Geometry check sheet. Reference: the model listing, model coordinates, mm. A direction names the side the tool comes from. Give positions to 0.01 mm unless a question says otherwise; leave off trailing zeros. Write each loop counter-clockwise with the first axis right and the second up, starting at its lowest first coordinate (ties: lowest second). Pieces come first, ordered by that corner, then holes. Notation, with made-up numbers: M 64.25,30.5 L 110.25,30.5 A33 ccw 110.25,58.5 Z; hole C -25.5,82.5 d2. An arc over 180 degrees is marked long. Write each question's results on one line, items separated by ' | '.
Autodesk Inventor part; units mm, degrees
ref_plane "YZ Plane" through (0, 0, 0) normal (1, 0, 0) x (0, 1, 0)
ref_plane "XZ Plane" through (0, 0, 0) normal (0, 1, 0) x (-1, 0, 0)
ref_plane "XY Plane" through (0, 0, 0) normal (0, 0, 1) x (1, 0, 0)
ref_plane "Work Plane1" through (0, 46.8, 0) normal (0, 0, 1) x (-1, 0, 0)
sketch "Sketch2" plane through (0, 46.8, 0) normal (0, 0, 1) x (-1, 0, 0)
  spline S0 degree 3 number of poles 148
  spline S1 degree 3 number of poles 148
  line L0 (31.3425, -5.6798) -> (32.5946, -4.8031)
  line L1 (32.5946, -4.1553) -> (31.3425, -3.2786)
  line L2 (31.3425, -3.2786) -> (31.3425, -5.6037)
  line L3 (32.5946, -4.8031) -> (32.5946, -4.1553)
  line L4 (31.3425, 13.5614) -> (31.3425, -5.6037)
  line L5 (32.8425, -4.1071) -> (31.4425, -3.1268)
  line L6 (31.4425, -3.1268) -> (31.4425, -2.831)
  line L7 (31.4425, -2.831) -> (32.8425, -1.8994)
  line L8 (32.8425, -1.8994) -> (32.8425, -4.1071)
  point P0 (0, 46.8)
  point P1 (31.9686, -3.7169)
  point P2 (32.1425, -3.6169)
  point P3 (31.4425, -2.9789)
  dimension "d4" = 0
  dimension "d5" = 0.1
  dimension "d6" = 0.1
  dimension "d7" = 1.4
coil "Coil1" sketch "Sketch2" operation add axis through (-23.4, 35.1998, 0) along (0, -1, 0) pitch 3 turns 2.5 hand right contours L5 L6 L7 L8
sketch "Sketch3" plane through (0, 46.8, 0) normal (0, 0, 1) x (-1, 0, 0)
  line L0 (13.9575, 5.6006) -> (13.9575, 3.3929)
  line L1 (32.8425, -1.8994) -> (32.8425, -4.1071)
  line L2 (15.3575, 4.669) -> (13.9575, 5.6006)
  line L3 (13.9575, 5.6006) -> (11.9575, 5.6006)
  line L4 (11.9575, 5.6006) -> (11.9575, -1.1071)
  line L5 (11.9575, -1.1071) -> (13.9575, -1.1071)
  line L6 (13.9575, -1.1071) -> (13.9575, 5.6006)
  line L7 (11.9575, -1.1071) -> (16.9575, -1.1071)
  line L8 (16.9575, -1.1071) -> (16.9575, -3.1071)
  line L9 (16.9575, -3.1071) -> (11.9575, -3.1071)
  line L10 (11.9575, -3.1071) -> (11.9575, -1.1071)
  line L11 (23.4, 56.7814) -> (23.4, -13.0885)
  point P0 (0, 46.8)
  dimension "d16" = 2
  dimension "d17" = 5
  dimension "d18" = 2
revolve "Revolution2" add sketch "Sketch3" angle 360 about axis through (-23.4, 35.1998, 0) along (0, 1, 0)
fillet "Fillet1" radius 1 4 edges at (-34.8425, 49.9071, 0) (-29.8425, 49.9071, 0) (-29.8425, 47.9071, 0) (-34.8425, 41.1994, 0)
properties part number "20_Cube_4_insert_Photosensor_lenscap"
Q1. Release check for a two-part mould opening along Z. For faces 3 (the face through (-34.83, 45.51, 0.5)), 4 (the face through (-29, 47.907, -6)), 5 (the face through (-32.3, 50.3, 0)), 6 (the face through (-20, 49.907, 7)) record: released by +Z, released by -Z, zero draft, split by the parting line, or undercut.
Answer key:
face 3: split by the parting line | face 4: undercut | face 5: released by +Z | face 6: zero draft
Q2. Material ranges on probe 1 along Z at (x, y) = (-23.4, 43); probe 2 along X at (y, z) = (48.95, 0); probe 3 along Y at (x, z) = (-20.5, 7), recorded low to high. Write a range as [from, to].
Answer key:
probe 1: z = [-11.44, -8.04], [9.44, 11.44] | probe 2: x = [-34.84, -29.84], [-16.96, -11.96] | probe 3: y = [47.91, 49.91]
Q3. Access from +Z, -Z, +X, -X, +Y, -Y to the whole of each face (thin tool, end or side, straight path). Record for faces 1 (the face through (-14.5, 42.3, 0)), 2 (the face through (-33, 41.199, 1)).
Answer key:
face 1: -Y | face 2: +Z, -Z, +X, -X, -Y
Q4. Section check A-A (y = 48.5). Enter the section's corners in (x, z) (1 decimal).
Answer key:
outline: C -23.4,0 d22.9; hole C -23.4,0 d13.1
Q5. Depth check by flat-ended pin: P1, Ø5, axis at y = 44, z = 5.5, coming from the +X side; P2, Ø1, axis at x = -28, y = 44.5, coming from the +Z side; P3, Ø10.5, axis at x = -24, z = -4.5, coming from the +Y side. Enter the tip coordinate at first touch or a pass-through.
Answer key:
P1: stops at x = -12.36 | P2: stops at z = 10.68 | P3: stops at y = 50.36
